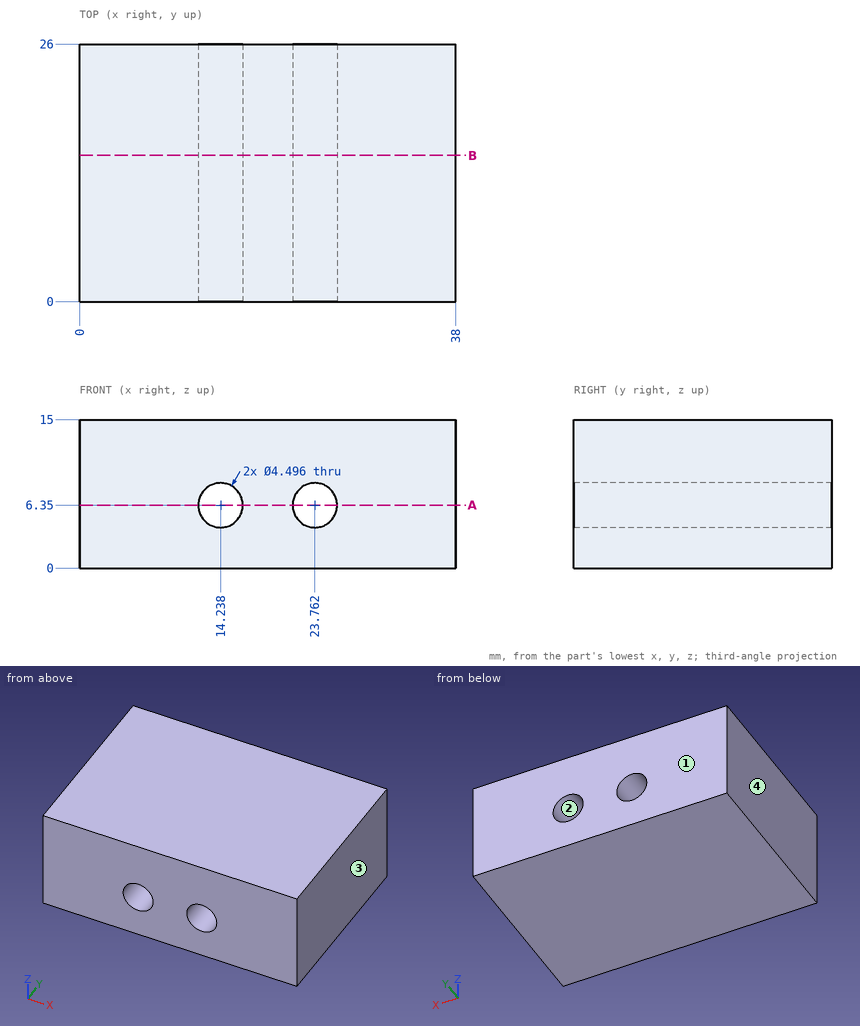
The figure shows three views and two pictorial views of one solid part (mm, origin at its lowest corner). Answer the questions. Round coordinates to 2 decimals unless told otherwise and drop trailing zeros. Loops run counter-clockwise (first coordinate to the right, second up) from the corner with the lowest first, then second, coordinate; pieces in that order, holes last. Notation, with made-up numbers: M 65,8 L 118,8 A16 ccw 118,24 Z; hole C -32.75,73 d8. An arc over 180 degrees is marked long. Return JSON: item names as keys, results as strings.
Q1. This flat-tipped pin is pushed along its axis until it touches: pin 1 Ø2 at (x, z) = (15, 11) entering from -Y. Where does it stop, or does it pass through?
Results list:
{"pin 1": "stops at y = 0"}
Q2. Find the intervals of material crossed by line 1 along X through (y, z) = (11, 5) (1 decimal); line 2 along X through (y, z) = (4.5, 4.75) (1 decimal); line 3 along Z through (x, y) = (24.5, 22.25) (1 decimal), in increasing order. Write a range as from..to.
Results list:
{"line 1": "x = 0..12.4, 16..22, 25.6..38", "line 2": "x = 0..12.7, 15.8..22.2, 25.3..38", "line 3": "z = 0..4.2, 8.5..15"}
Q3. Find section A-A, the plane z = 6.35. Determine the outline of the cut face in (x, y) (1 decimal), plus the area to 3 significant figures.
Results list:
{"outline": "M 0,0 L 12,0 L 12,26 L 0,26 Z; M 16.5,0 L 21.5,0 L 21.5,26 L 16.5,26 Z; M 26,0 L 38,0 L 38,26 L 26,26 Z", "area": "754 mm2"}
Q4. Find section B-B, the plane y = 14.75. State how many separate pieces and enclosed holes the cut face has, plus the area to 3 significant figures.
Results list:
{"separate pieces": "1", "enclosed holes": "2", "area": "538 mm2"}
Q5. The mould has two halves that part along X. Classify the marked faces 1, 2, 3 and 4: released by +X, released by -X, zero draft, split by the parting line, or undercut.
Results list:
{"face 1": "zero draft", "face 2": "undercut", "face 3": "released by +X", "face 4": "released by -X"}
